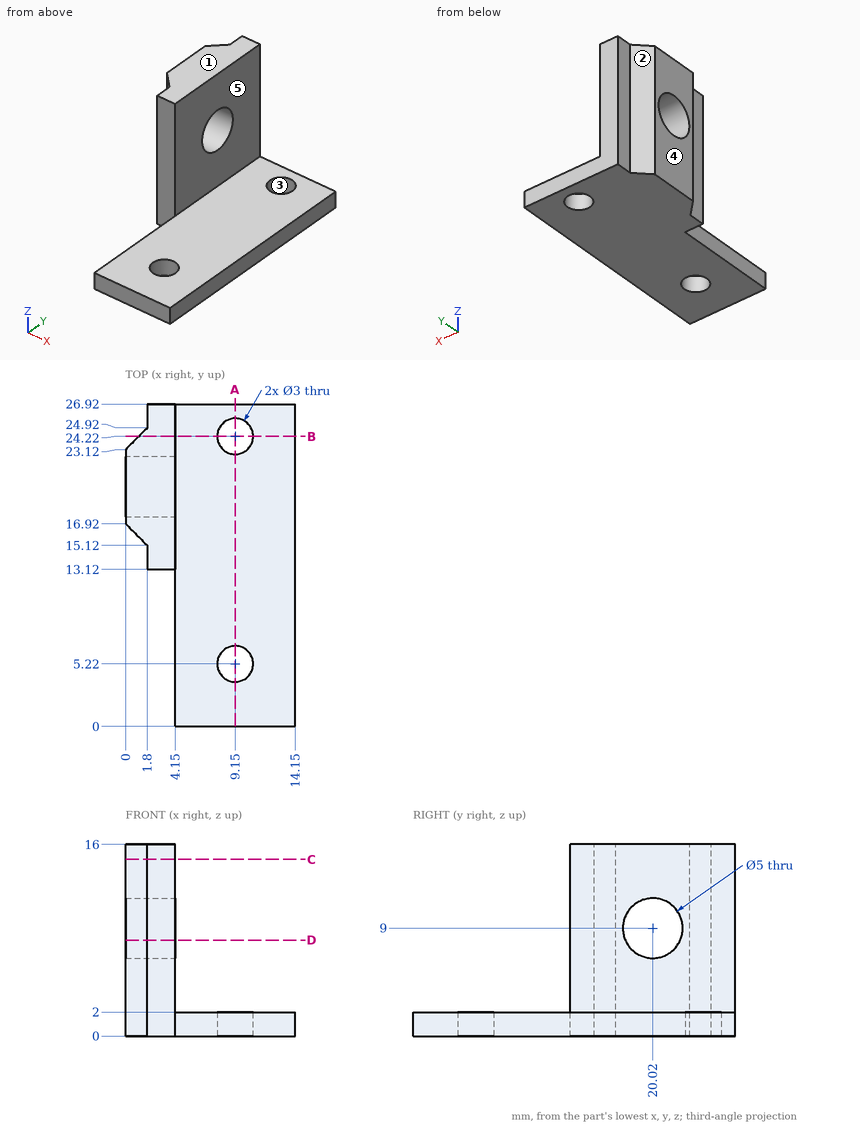
Geometry check sheet. Reference: drawing and pictorial views, mm from the part's lowest x, y, z. A direction names the side the tool comes from. Round coordinates to 2 decimals unless told otherwise and drop trailing zeros. Order: outer loops, then holes, each group sorted by start corner. A loop starts at its lowest first (then second) coordinate and runs counter-clockwise, first axis right, second up. Notation, with made-up numbers: M 49.5,-29 L 81.5,-29 A24 cw 81.5,0 Z; hole C -2,38.5 d10. An arc over 180 degrees is marked long. One line per item, written item: value. Start each with the question number.
1. Section check B-B on y = 24.22. Enter the section's corners in (x, z), and give its area (3 significant figures).
2. Section check D-D on z = 8. Enter the section's corners in (x, y), and give its area (3 significant figures).
3. Section check A-A on x = 9.15. Enter the section's corners in (y, z), and give its area (3 significant figures).
4. Section check C-C on z = 14.75. Enter the section's corners in (x, y).
5. Release check for a two-part mould opening along X. For the marked faces 1, 2 and 3 record: released by +X, released by -X, zero draft, split by the parting line, or undercut.
6. Access from +Z, -Z, +X, -X, +Y, -Y to the whole of each face (thin tool, end or side, straight path). Record for the marked faces 4 and 5.
7. Gauge pin test, flat ends, axial feed: P1, Ø1.5, axis at x = 9, y = 10.5, coming from the +Z side; P2, Ø0.7, axis at x = 2.5, z = 6, coming from the -Y side; P3, Ø1.8, axis at x = 9.15, y = 24.22, coming from the -Z side; P4, Ø2, axis at y = 14.5, z = 6.5, coming from the -X side. Record the tip position at first contact, or that the pin passes through.
8. Scan lines: line 1 along Y through (x, z) = (9.15, 0.8); line 2 along Z through (x, y) = (11.5, 6.5); line 3 along X through (y, z) = (18.75, 15.5). Record each from-to range of solid material in increasing order.
Results found:
1. outline: M 1.1,0 L 7.65,0 L 7.65,2 L 4.15,2 L 4.15,16 L 1.1,16 Z; M 10.65,0 L 14.15,0 L 14.15,2 L 10.65,2 Z
1. area: 62.8 mm^2
2. outline: M 0,16.92 L 1.8,15.12 L 1.8,13.12 L 4.15,13.12 L 4.15,17.73 L 0,17.73 Z; M 0,22.31 L 4.15,22.31 L 4.15,26.92 L 1.8,26.92 L 1.8,24.92 L 0,23.12 Z
2. area: 27.8 mm^2
3. outline: M 0,0 L 3.72,0 L 3.72,2 L 0,2 Z; M 6.72,0 L 22.72,0 L 22.72,2 L 6.72,2 Z; M 25.72,0 L 26.92,0 L 26.92,2 L 25.72,2 Z
3. area: 41.8 mm^2
4. outline: M 0,16.92 L 1.8,15.12 L 1.8,13.12 L 4.15,13.12 L 4.15,26.92 L 1.8,26.92 L 1.8,24.92 L 0,23.12 Z
5. face 1: zero draft
5. face 2: released by -X
5. face 3: undercut
6. face 4: +Z, -Z, -X, +Y, -Y
6. face 5: +Z, +X, +Y, -Y
7. P1: z = 2
7. P2: y = 13.12
7. P3: through
7. P4: x = 1.42
8. line 1: 0 to 3.72, 6.72 to 22.72, 25.72 to 26.92
8. line 2: 0 to 2
8. line 3: 0 to 4.15
